Here's how the part is built. I have some questions about the finished solid (model axes, mm). Round coordinates to 2 decimals unless told otherwise and drop trailing zeros. Loops run counter-clockwise (first coordinate to the right, second up) from the corner with the lowest first, then second, coordinate; pieces in that order, holes last. Notation, with made-up numbers: M -17,67.25 L 5,67.25 A11 ccw 5,75.25 Z; hole C 26.25,64 d2. An arc over 180 degrees is marked long. Use a Markdown table: item, result.
from build123d import *

# Parameters (mm, degrees)
DODANIE_WYCI_GNI_CIE1_DEPTH = 580


with BuildPart() as part:
    # Szkic1 → Dodanie-wyciągnięcie1 (new body)
    with BuildSketch(Plane.XY):
        with BuildLine():
            Line((-3.487119155, 17.8), (-8.605626905, 11.7))
            Line((-8.605626905, 11.7), (-9.25, 11.7))
            Line((-9.25, 11.7), (-9.25, 5))
            Line((-9.25, 5), (-20, 5))
            Line((-20, 5), (-20, 0))
            Line((-20, 0), (-8.605626905, 0))
            Line((-8.605626905, 0), (-7.766527274, 1))
            Line((-7.766527274, 1), (7.766527274, 1))
            Line((7.766527274, 1), (8.605626905, 0))
            Line((8.605626905, 0), (20, 0))
            Line((20, 0), (20, 5))
            Line((20, 5), (9.25, 5))
            Line((9.25, 5), (9.25, 11.7))
            Line((9.25, 11.7), (8.605626905, 11.7))
            Line((8.605626905, 11.7), (3.487119155, 17.8))
            ThreePointArc((3.487119155, 17.8), (0, 33), (-3.487119155, 17.8))
        make_face()
    extrude(amount=DODANIE_WYCI_GNI_CIE1_DEPTH)


solid = part.part
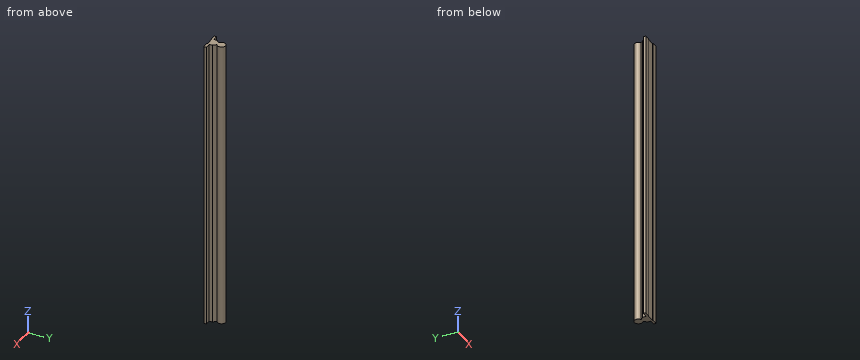
1. I need wall thicknesses on probe 1 along X at (y, z) = (6.5, 231); probe 2 along Y at (x, z) = (17.5, 232); probe 3 along Y at (x, z) = (1, 256). Which ranges of each line are inside material? Lowest first, please. Write a range as from..to.
Answer sheet:
| item | result |
|---|---|
| probe 1 | -9.25..9.25 |
| probe 2 | 0..5 |
| probe 3 | 1..32.94 |
2. For pin 1 Ø3 at (y, z) = (13.5, 252) entering from -X; pin 2 Ø2 at (y, z) = (7.5, 161) entering from -X; pin 3 Ø3 at (x, z) = (12, 179.5) entering from +Y, each with a flat end and sliding along its axis, tell me the tip position at first contact or that it passes through.
Answer sheet:
| item | result |
|---|---|
| pin 1 | x = -8.35 |
| pin 2 | x = -9.25 |
| pin 3 | y = 5 |
3. Imagine slicing it at B-B, the plane y = 25. Write out the boundary of the cut face in (x, z), then the cut area to 3 significant figures.
Answer sheet:
| item | result |
|---|---|
| outline | M -8,0 L 8,0 L 8,580 L -8,580 Z |
| area | 9,280 mm2 |
4. Imagine slicing it at A-A, the plane z = 224. Write out the boundary of the cut face in (x, y), then the cut area to 3 significant figures.
Answer sheet:
| item | result |
|---|---|
| outline | M -20,0 L -8.61,0 L -7.77,1 L 7.77,1 L 8.61,0 L 20,0 L 20,5 L 9.25,5 L 9.25,11.7 L 8.61,11.7 L 3.49,17.8 A8 ccw long -3.49,17.8 L -8.61,11.7 L -9.25,11.7 L -9.25,5 L -20,5 Z |
| area | 579 mm2 |
